Job drawing, mm, ordinate dimensions from the low corner. One solid piece. Coordinates: 2 decimals unless noted, no trailing zeros. Write each loop counter-clockwise with the first axis right and the second up, starting at its lowest first coordinate (ties: lowest second). Pieces come first, ordered by that corner, then holes. Notation, with made-up numbers: (32.5, -3) -> (39.5, -3) arc R27 cw to (39.5, 35) -> close; hole circle Ø6 at (67, -25.75). An arc over 180 degrees is marked (long way). Answer as a JSON object with one key per item and string values. Group by question number.
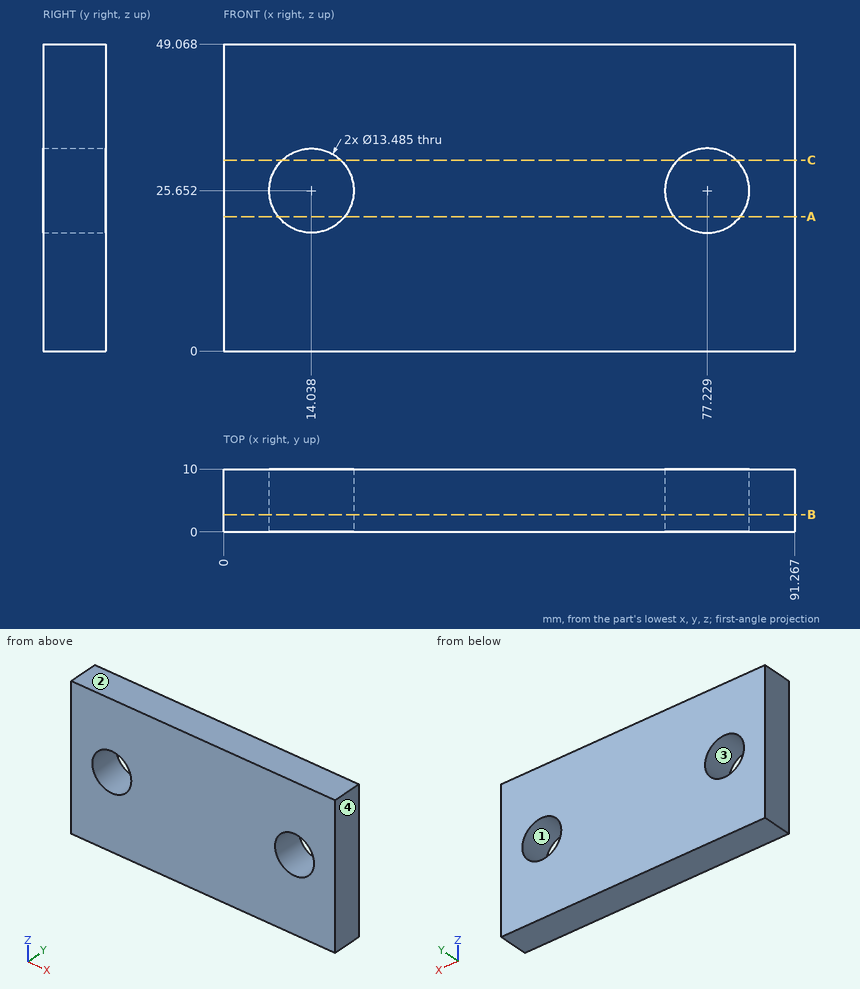
(1) Cut at B-B on y = 2.75. List the corners of the cut face in (x, z) (1 decimal), plus the area to 3 significant figures.
(2) Cut at C-C on z = 30.5. List the corners of the cut face in (x, y) (1 decimal), plus the area to 3 significant figures.
(3) Wall check: probe 1 along X at (y, z) = (8.75, 26) (1 decimal); probe 2 along X at (y, z) = (6, 24.5) (1 decimal); probe 3 along Z at (x, y) = (14, 7.75) (1 decimal). Give the ranges that are in metal, low to high.
(4) Pull direction X, two halves, no side cores. Call the marked faces 1, 2, 3 and 4: released by +X, released by -X, zero draft, split by the parting line, or undercut.
(5) Cut at A-A on z = 21.5. Give the number of separate pieces and of enclosed holes in the cut face, plus the area to 3 significant figures.
Results found:
{
 "1": {"outline": "(0, 0) -> (91.3, 0) -> (91.3, 49.1) -> (0, 49.1) -> close; hole circle Ø13.5 at (14, 25.7); hole circle Ø13.5 at (77.2, 25.7)", "area": "4,190 mm²"},
 "2": {"outline": "(0, 0) -> (9.4, 0) -> (9.4, 10) -> (0, 10) -> close; (18.7, 0) -> (72.5, 0) -> (72.5, 10) -> (18.7, 10) -> close; (81.9, 0) -> (91.3, 0) -> (91.3, 10) -> (81.9, 10) -> close", "area": "725 mm²"},
 "3": {"probe 1": "x = 0 to 7.3, 20.8 to 70.5, 84 to 91.3", "probe 2": "x = 0 to 7.4, 20.7 to 70.6, 83.9 to 91.3", "probe 3": "z = 0 to 18.9, 32.4 to 49.1"},
 "4": {"face 1": "undercut", "face 2": "zero draft", "face 3": "undercut", "face 4": "released by +X"},
 "5": {"separate pieces": "3", "enclosed holes": "0", "area": "700 mm²"}
}
